from build123d import *

# Parameters (mm, degrees)
SKETCH1_R           = 5
BOSS_EXTRUDE1_DEPTH = 10
SKETCH2_R           = 5
BOSS_EXTRUDE2_DEPTH = 15
SKETCH3_W           = 5
SKETCH3_H           = 260
BOSS_EXTRUDE3_DEPTH = 35
SKETCH8_W           = 5
SKETCH8_H           = 19
BOSS_EXTRUDE4_DEPTH = 20
SKETCH9_W           = 19
SKETCH9_H           = 10
SKETCH9_H_2         = 20
BOSS_EXTRUDE5_DEPTH = 45
SKETCH10_W          = 19
SKETCH10_H          = 40
BOSS_EXTRUDE6_DEPTH = 10
BOSS_EXTRUDE7_DEPTH = 5
SKETCH12_W          = 40
SKETCH12_H          = 30
CUT_EXTRUDE1_DEPTH  = 10


with BuildPart() as part:
    # Sketch1 → Boss-Extrude1 (new body)
    with BuildSketch(Plane.XY):
        with BuildLine():
            Line((-5, -20), (5, -20))
            ThreePointArc((5, -20), (19.142135624, -14.142135624), (25, 0))
            Line((25, 0), (25, 260))
            ThreePointArc((25, 260), (19.142135624, 274.142135624), (5, 280))
            Line((5, 280), (-5, 280))
            ThreePointArc((-5, 280), (-19.142135624, 274.142135624), (-25, 260))
            Line((-25, 260), (-25, 0))
            ThreePointArc((-25, 0), (-19.142135624, -14.142135624), (-5, -20))
        make_face()
        Circle(SKETCH1_R, mode=Mode.SUBTRACT)
    boss_extrude1 = extrude(amount=BOSS_EXTRUDE1_DEPTH)

    # Sketch2 → Boss-Extrude2 (add)
    with BuildSketch(Plane.XY.offset(10)):
        with Locations((0, 260)):
            Circle(SKETCH2_R)
    boss_extrude2 = extrude(amount=BOSS_EXTRUDE2_DEPTH)

    # Sketch3 → Boss-Extrude3 (add)
    with BuildSketch(Plane(origin=(0, 0, 0), x_dir=(-1, 0, 0), z_dir=(0, 0, -1))):
        with Locations((22.5, 130)):
            Rectangle(SKETCH3_W, SKETCH3_H)
    boss_extrude3 = extrude(amount=BOSS_EXTRUDE3_DEPTH)

    # Mirror1: Boss-Extrude1, Boss-Extrude2, Boss-Extrude3 across plane
    add(boss_extrude1.mirror(Plane.XY.offset(-35)))
    add(boss_extrude2.mirror(Plane.XY.offset(-35)))
    add(boss_extrude3.mirror(Plane.XY.offset(-35)))

    # Sketch8 → Boss-Extrude4 (add)
    with BuildSketch(Plane.XZ):
        with Locations((-22.5, -39.5)):
            Rectangle(SKETCH8_W, SKETCH8_H)
    extrude(amount=BOSS_EXTRUDE4_DEPTH)

    # Sketch9 → Boss-Extrude5 (add)
    with BuildSketch(Plane(origin=(-20, 0, 0), x_dir=(0, 0, -1), z_dir=(1, 0, 0))):
        with Locations((39.5, -15)):
            Rectangle(SKETCH9_W, SKETCH9_H)
        with Locations((39.5, 40)):
            Rectangle(SKETCH9_W, SKETCH9_H_2)
    extrude(amount=BOSS_EXTRUDE5_DEPTH)

    # Sketch10 → Boss-Extrude6 (add)
    with BuildSketch(Plane(origin=(-20, 0, 0), x_dir=(0, 0, -1), z_dir=(1, 0, 0))):
        with Locations((39.5, 10)):
            Rectangle(SKETCH10_W, SKETCH10_H)
    extrude(amount=BOSS_EXTRUDE6_DEPTH)

    # Sketch11 → Boss-Extrude7 (add)
    with BuildSketch(Plane.ZY.offset(25)):
        Polygon((10, 0), (-30, 0), (-30, -20), (-49, -20), (-49, 0), (-80, 0), (-80, 260), (10, 260), align=None)
    extrude(amount=BOSS_EXTRUDE7_DEPTH)

    # Sketch12 → Cut-Extrude1 (cut)
    with BuildSketch(Plane.ZY.offset(30)):
        with Locations((-35, 245)):
            Rectangle(SKETCH12_W, SKETCH12_H)
    extrude(amount=-CUT_EXTRUDE1_DEPTH, mode=Mode.SUBTRACT)


solid = part.part
Source: CAD feature listing. Evaluate the final solid. Frame: model axes, mm. A direction names the side the tool comes from. Coordinates: 2 decimals unless noted, no trailing zeros. Write each loop counter-clockwise with the first axis right and the second up, starting at its lowest first coordinate (ties: lowest second). Pieces come first, ordered by that corner, then holes. Notation, with made-up numbers: M 28,62 L 75,62 A24 ccw 75,100 Z; hole C 67.25,45.5 d8. An arc over 180 degrees is marked long. Use a Markdown table: item, result.
1) First-contact query: pin 1 Ø1 at (y, z) = (40, -6.5) entering from +X; pin 2 Ø8 at (x, z) = (-23, -38.5) entering from +Y; pin 3 Ø4 at (x, y) = (-11, 211.5) entering from +Z. Flat tips, straight axial feed; report the tip coordinate or a pass-through.
Conclusion:
| item | result |
|---|---|
| pin 1 | stops at x = -20 |
| pin 2 | stops at y = 230 |
| pin 3 | stops at z = 10 |
2) Section B-B, the plane y = 33.5. Output: boundary loops of the cut face in (x, z), then the cut area to 4 significant figures.
Conclusion:
| item | result |
|---|---|
| outline | M -30,-80 L 25,-80 L 25,-70 L -20,-70 L -20,-49 L 25,-49 L 25,-30 L -20,-30 L -20,0 L 25,0 L 25,10 L -30,10 Z |
| area | 2,655 mm^2 |
3) Reachability of faces 1 (the cylindrical face through (18.986, -14.297, -74.93)), 2 (the cylindrical face through (18.986, -14.297, 4.93)), 3 (the cylindrical face through (-19.297, -13.986, 4.93)), 4 (the cylindrical face through (-19.297, -13.986, -74.93)), 5 (the cylindrical face through (-0.651, 264.957, 17.395)) from +Z, -Z, +X, -X, +Y, -Y: full face, straight path, thin tool, end or side. Return the list, or none.
Conclusion:
| item | result |
|---|---|
| face 1 | -Z, +X, -Y |
| face 2 | +Z, +X, -Y |
| face 3 | +Z, -X, -Y |
| face 4 | -Z, -X, -Y |
| face 5 | +Z |
4) Section A-A, the plane z = -39.5. Output: boundary loops of the cut face in (x, y).
Conclusion:
| item | result |
|---|---|
| outline | M -30,-20 L 25,-20 L 25,-10 L -10,-10 L -10,30 L 25,30 L 25,50 L -20,50 L -20,230 L -30,230 Z |
5) Mould query, pull axis X, two halves, no side actions, for faces 6 (the cylindrical face through (-1.08, -4.88, 4.93)), 7 (the flat face through (-2, 132, 10)), 8 (the flat face through (25, 128, -75)). Classes: pulls with the +X half, pulls with the -X half, needs draft (parallel to the pull), parting line crosses it, or undercut.
Conclusion:
| item | result |
|---|---|
| face 6 | undercut |
| face 7 | needs draft |
| face 8 | pulls with the +X half |
6) Ray query, L1, parallel to Z at x = -2, y = 34; L2, parallel to Y at x = 19, z = -41; L3, parallel to Z at x = -19, y = 110. Return the intervals inside material, ascending.
Conclusion:
| item | result |
|---|---|
| L1 | z = -80 to -70, -49 to -30, 0 to 10 |
| L2 | y = -20 to -10, 30 to 50 |
| L3 | z = -80 to -70, 0 to 10 |
7) Section D-D, the plane z = -77. Output: boundary loops of the cut face in (x, y).
Conclusion:
| item | result |
|---|---|
| outline | M -30,0 L -25,0 A20 ccw -5,-20 L 5,-20 A20 ccw 25,0 L 25,260 A20 ccw 5,280 L -5,280 A20 ccw -25,260 L -30,260 Z; hole C 0,0 d10 |
8) Section C-C, the plane x = 16.5. Output: boundary loops of the cut face in (y, z).
Conclusion:
| item | result |
|---|---|
| outline | M -20,-49 L -10,-49 L -10,-30 L -20,-30 Z; M -16.36,-80 L 276.36,-80 L 276.36,-70 L -16.36,-70 Z; M -16.36,0 L 276.36,0 L 276.36,10 L -16.36,10 Z; M 30,-49 L 50,-49 L 50,-30 L 30,-30 Z |
